Read the model definition and answer for the solid it produces. Units are mm, in the model's axes. Coordinates: 2 decimals unless noted, no trailing zeros. Write each loop counter-clockwise with the first axis right and the second up, starting at its lowest first coordinate (ties: lowest second). Pieces come first, ordered by that corner, then holes. Notation, with made-up numbers: M 12,73.25 L 40,73.25 A21 ccw 40,106.25 Z; hole C -32.75,-40 d9. An arc over 180 degrees is marked long. Write item = value, one per line.
from build123d import *

# Parameters (mm, degrees)
BOSS_EXTRUDE1_DEPTH = 1.00076
SKETCH2_W           = 2.472118206
SKETCH2_H           = 1.00076
BOSS_EXTRUDE2_DEPTH = 3.175
CHAMFER2_SIZE       = 19.05
CHAMFER3_SIZE       = 3.175


with BuildPart() as part:
    # Sketch1 → Boss-Extrude1 (new body)
    with BuildSketch(Plane(origin=(0, 0, 0), x_dir=(1, 0, 0), z_dir=(0, 1, 0))):
        Polygon((-3.175, -41.275), (-3.175, -47.625), (-12.7, -47.625), (-12.7, -57.15), (12.7, -57.15), (12.7, -41.275), (12.7, 41.275), (-12.7, 41.275), (-12.7, -41.275), align=None)
    extrude(amount=BOSS_EXTRUDE1_DEPTH)

    # Sketch2 → Boss-Extrude2 (add)
    with BuildSketch(Plane.XY.offset(41.275)):
        with Locations((-11.463940897, 0.50038)):
            Rectangle(SKETCH2_W, SKETCH2_H)
    boss_extrude2 = extrude(amount=BOSS_EXTRUDE2_DEPTH)

    # Mirror1: Boss-Extrude2 across plane
    add(boss_extrude2.mirror(Plane.XY))

    # Chamfer2
    chamfer2_edges = [part.edges().sort_by_distance(p)[0] for p in [
        (12.7, 0.50038, 57.15),
    ]]
    chamfer(chamfer2_edges, length=CHAMFER2_SIZE)

    # Chamfer3
    chamfer3_edges = [part.edges().sort_by_distance(p)[0] for p in [
        (-3.175, 0.50038, 47.625),
    ]]
    chamfer(chamfer3_edges, length=CHAMFER3_SIZE)


solid = part.part
Item 1: Find section C-C (x = 4.25). Determine the outline of the cut face in (y, z) (3 decimals), and give its area (3 significant figures).
Worked answers:
outline = M 0,-41.275 L 1.001,-41.275 L 1.001,46.55 L 0,46.55 Z
area = 87.9 mm²
Item 2: A flat-ended cylindrical pin translates along its axis: pin 1 (0.5 mm diameter, centred on y = 0.5, z = 43, fed in from +X). Find the tip coordinate at first contact, or state that the pin passes through.
Worked answers:
pin_1 = 8.05
Item 3: Find section A-A (y = 0.7). Determine the outline of the cut face in (x, z) (3 decimals).
Worked answers:
outline = M -12.7,-44.45 L -10.228,-44.45 L -10.228,-41.275 L 12.7,-41.275 L 12.7,38.1 L -6.35,57.15 L -12.7,57.15 L -12.7,47.625 L -6.35,47.625 L -3.175,44.45 L -3.175,41.275 L -10.228,41.275 L -10.228,44.45 L -12.7,44.45 Z
Item 4: Find section D-D (x = 11). Determine the outline of the cut face in (y, z) (3 decimals).
Worked answers:
outline = M 0,-41.275 L 1.001,-41.275 L 1.001,39.8 L 0,39.8 Z
Item 5: Find section B-B (x = -4.5). Determine the outline of the cut face in (y, z) (3 decimals), and give its area (3 significant figures).
Worked answers:
outline = M 0,-41.275 L 1.001,-41.275 L 1.001,41.275 L 0,41.275 Z; M 0,45.775 L 1.001,45.775 L 1.001,55.3 L 0,55.3 Z
area = 92.1 mm²
Item 6: Consider line 1 along Z through (x, y) = (-11, 0.5) (3 decimals); line 2 along Z through (x, y) = (-8.75, 0.9) (3 decimals); line 3 along Z through (x, y) = (1, 0.8) (3 decimals). Determine where each line is inside the solid, lowest interval first. Write a range as from..to.
Worked answers:
line_1 = -44.45..44.45, 47.625..57.15
line_2 = -41.275..41.275, 47.625..57.15
line_3 = -41.275..49.8
